```python
from build123d import *

# Parameters (mm, degrees)
SKETCH_1_R          = 2.15
SKETCH_1_R_2        = 12
SKETCH_1_R_3        = 3
SKETCH_1_R_4        = 2.1
EXTRUDE_1_DEPTH     = 3
CUT_EXTRUDE_1_DEPTH = 3
FILLET_1_R          = 2
FILLET_2_R          = 2
FILLET_3_R          = 3


with BuildPart() as part:
    # ｽｹｯﾁ1 → ﾎﾞｽ - 押し出し1 (new body)
    with BuildSketch(Plane(origin=(0, 0, 0), x_dir=(0, 0, -1), z_dir=(1, 0, 0))):
        with BuildLine():
            Line((0, 0), (20, 0))
            Line((20, 0), (81.721631315, 15.55153458))
            ThreePointArc((81.721631315, 15.55153458), (83.805915962, 16.648877548), (85.156498305, 18.57873024))
            ThreePointArc((85.156498305, 18.57873024), (91.240951268, 28.202978223), (100.473591964, 34.86669062))
            ThreePointArc((100.473591964, 34.86669062), (101.625387424, 35.607613327), (102.53294649, 36.633252532))
            ThreePointArc((102.53294649, 36.633252532), (109.848876527, 44.266796828), (119.358709974, 48.888149295))
            ThreePointArc((119.358709974, 48.888149295), (121.530071674, 50.159012288), (122.807632728, 52.326439826))
            Line((122.807632728, 52.326439826), (125, 60))
            Line((125, 60), (125, 70))
            Line((125, 70), (106.736076333, 88.580227744))
            ThreePointArc((106.736076333, 88.580227744), (105.828986144, 89.309735766), (104.777796911, 89.809731531))
            ThreePointArc((104.777796911, 89.809731531), (92.392887273, 97.853140314), (85.346092725, 110.831009869))
            ThreePointArc((85.346092725, 110.831009869), (84.032111964, 113.138952539), (81.721631315, 114.44846542))
            Line((81.721631315, 114.44846542), (20, 130))
            Line((20, 130), (0, 130))
            Line((0, 130), (0, 0))
        make_face()
        with Locations((7.5, 120)):
            Circle(SKETCH_1_R, mode=Mode.SUBTRACT)
        with Locations((7.5, 90)):
            Circle(SKETCH_1_R, mode=Mode.SUBTRACT)
        with Locations(Location((7.5, 40, 0), (0, 0, 180))):
            Circle(SKETCH_1_R, mode=Mode.SUBTRACT)
        with Locations(Location((7.5, 10, 0), (0, 0, 180))):
            Circle(SKETCH_1_R, mode=Mode.SUBTRACT)
        with Locations((74.5, 65)):
            Circle(SKETCH_1_R_2, mode=Mode.SUBTRACT)
        with Locations((29.5, 65)):
            Circle(SKETCH_1_R_3, mode=Mode.SUBTRACT)
        with Locations((80.5, 20.4)):
            Circle(SKETCH_1_R_3, mode=Mode.SUBTRACT)
        with Locations((118, 53.7)):
            Circle(SKETCH_1_R_3, mode=Mode.SUBTRACT)
        with Locations((80.5, 109.6)):
            Circle(SKETCH_1_R_3, mode=Mode.SUBTRACT)
        with Locations((103.17032155, 85.075175272)):
            Circle(SKETCH_1_R, mode=Mode.SUBTRACT)
        with Locations((98.369942602, 39.402620443)):
            Circle(SKETCH_1_R, mode=Mode.SUBTRACT)
        with Locations((105, 65)):
            Circle(SKETCH_1_R, mode=Mode.SUBTRACT)
        with Locations((120, 65)):
            Circle(SKETCH_1_R, mode=Mode.SUBTRACT)
        with Locations((25, 12)):
            Circle(SKETCH_1_R_4, mode=Mode.SUBTRACT)
        with Locations((50.4, 12)):
            Circle(SKETCH_1_R_4, mode=Mode.SUBTRACT)
    extrude(amount=EXTRUDE_1_DEPTH)

    # ｽｹｯﾁ2 → ｶｯﾄ - 押し出し1 (cut)
    with BuildSketch(Plane(origin=(3, 0, 0), x_dir=(0, 0, -1), z_dir=(1, 0, 0))):
        with BuildLine():
            Line((20, 114.531188015), (20, 72.399324293))
            ThreePointArc((20, 72.399324293), (27.112840869, 92.918759813), (41.614001532, 109.085270837))
            Line((41.614001532, 109.085270837), (20, 114.531188015))
        make_face()
        with BuildLine():
            Line((20, 15.468811985), (41.614001532, 20.914729163))
            ThreePointArc((41.614001532, 20.914729163), (27.112840869, 37.081240187), (20, 57.600675707))
            Line((20, 57.600675707), (20, 15.468811985))
        make_face()
    extrude(amount=-CUT_EXTRUDE_1_DEPTH, mode=Mode.SUBTRACT)

    # ﾌｨﾚｯﾄ1
    fillet_1_edges = [part.edges().sort_by_distance(p)[0] for p in [
        (1.5, 130, 0),
        (1.5, 130, -20),
        (1.5, 0, -20),
        (1.5, 0, 0),
    ]]
    fillet(fillet_1_edges, radius=FILLET_1_R)

    # ﾌｨﾚｯﾄ2
    fillet_2_edges = [part.edges().sort_by_distance(p)[0] for p in [
        (1.5, 70, -125),
        (1.5, 60, -125),
    ]]
    fillet(fillet_2_edges, radius=FILLET_2_R)

    # ﾌｨﾚｯﾄ3
    fillet_3_edges = [part.edges().sort_by_distance(p)[0] for p in [
        (1.5, 114.531188015, -20),
        (1.5, 109.085270837, -41.614001532),
        (1.5, 72.399324293, -20),
        (1.5, 15.468811985, -20),
        (1.5, 57.600675707, -20),
        (1.5, 20.914729163, -41.614001532),
    ]]
    fillet(fillet_3_edges, radius=FILLET_3_R)


solid = part.part
```
The listing builds one solid part. Answer for the finished solid, in the listing's coordinates (mm). A direction names the side the tool comes from. Round coordinates to 2 decimals unless told otherwise and drop trailing zeros. Write each loop counter-clockwise with the first axis right and the second up, starting at its lowest first coordinate (ties: lowest second). Pieces come first, ordered by that corner, then holes. Notation, with made-up numbers: (50.25, 7.5) -> (67.25, 7.5) arc R31 ccw to (67.25, 39.5) -> close; hole circle Ø5 at (79, 57.5). An arc over 180 degrees is marked (long way). Use CSV: the item, a comma, the result in double quotes. Start each with the question number.
(1) Consider L1, parallel to Y at x = 1.95, z = -7.5; L2, parallel to Z at x = 2.4, y = 91; L3, parallel to Y at x = 2, z = -79.5. Determine where each line is inside the solid, lowest interval first. Write a range as from..to.
(2) Section B-B on y = 32 is taken. Give the vertices of the cut face in (x, z), then the cut area to 3 significant figures.
(3) The mould has two halves that part along Z. Classify faces 1 (the face through (1.479, 97.7, -92.535)), 2 (the face through (1.479, 64.177, -121.986)), 3 (the face through (3, 66, -48)), 4 (the face through (1.52, 98.25, -30.69)): released by +Z, released by -Z, zero draft, split by the parting line, or undercut.
(4) Each of these flat-tipped pins is pushed along its axis until it touches: pin 1 (3.5 mm diameter, centred on y = 65, z = -120, fed in from -X); pin 2 (1 mm diameter, centred on x = 2, y = 93.5, fed in from -Z); pin 3 (1.5 mm diameter, centred on x = 2, y = 30.5, fed in from -Z); pin 4 (1 mm diameter, centred on x = 0.5, z = -22, fed in from -Y). Where does it stop, or does it pass through?
(5) Section C-C on z = -74.5 is taken. Give the vertices of the cut face in (x, y), then the cut area to 3 significant figures.
(6) Section D-D on x = 1.8 is taken. Count the separate pieces of the cut face and the enclosed holes in it, then the cut area to 3 significant figures.
(7) Section A-A on z = -7.5 is taken. Give the vertices of the cut face in (x, y), then the cut area to 3 significant figures.
(8) Which of the six approach directions +Z, -Z, +X, -X, +Y, -Y give full straight-line access (tool end or side, diameter ignored) to faces 5 (the face through (1, 130, -11)), 6 (the face through (1.479, 41.249, -22.344))?
A:
1,L1,"y = 0..7.85, 12.15..37.85, 42.15..87.85, 92.15..117.85, 122.15..130"
1,L2,"z = -101.8..-26.03, -20.08..-9.4, -5.6..0"
1,L3,"y = 14.99..17.57, 23.23..54.09, 75.91..106.77, 112.43..115.01"
2,outline,"(0, -95.57) -> (3, -95.57) -> (3, -30.5) -> (0, -30.5) -> close; (0, -20) -> (3, -20) -> (3, 0) -> (0, 0) -> close"
2,area,"255 mm²"
3,face 1,"released by -Z"
3,face 2,"undercut"
3,face 3,"zero draft"
3,face 4,"undercut"
4,pin 1,"passes through"
4,pin 2,"stops at z = -98.17"
4,pin 3,"stops at z = -94.57"
4,pin 4,"stops at y = 0.38"
5,outline,"(0, 13.73) -> (3, 13.73) -> (3, 53) -> (0, 53) -> close; (0, 77) -> (3, 77) -> (3, 116.27) -> (0, 116.27) -> close"
5,area,"236 mm²"
6,separate pieces,"1"
6,enclosed holes,"17"
6,area,"10,700 mm²"
7,outline,"(0, 0) -> (3, 0) -> (3, 7.85) -> (0, 7.85) -> close; (0, 12.15) -> (3, 12.15) -> (3, 37.85) -> (0, 37.85) -> close; (0, 42.15) -> (3, 42.15) -> (3, 87.85) -> (0, 87.85) -> close; (0, 92.15) -> (3, 92.15) -> (3, 117.85) -> (0, 117.85) -> close; (0, 122.15) -> (3, 122.15) -> (3, 130) -> (0, 130) -> close"
7,area,"338 mm²"
8,face 5,"+Z, -Z, +X, -X, +Y"
8,face 6,"+X, -X"
